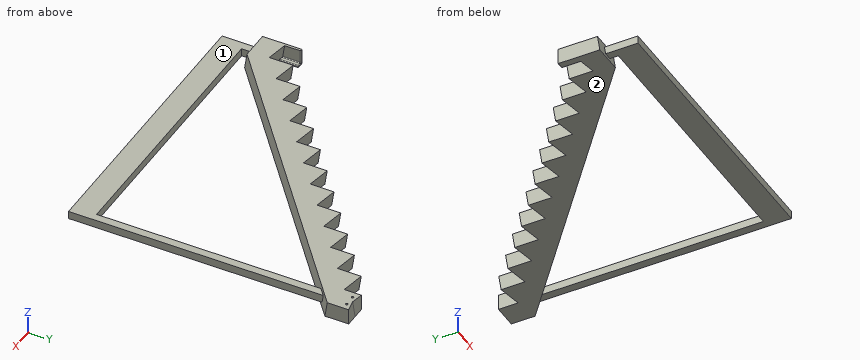
```python
from build123d import *

# Parameters (mm, degrees)
BOSS_EXTRUDE3_DEPTH      = 20
BOSS_EXTRUDE3_DEPTH_BACK = 13
FILLET2_R                = 1
BOSS_EXTRUDE4_DEPTH      = 20
BOSS_EXTRUDE4_DEPTH_BACK = 40
SKETCH10_W               = 10
SKETCH10_H               = 10
BOSS_EXTRUDE5_DEPTH      = 300
BOSS_EXTRUDE5_DEPTH_BACK = 40
SKETCH12_W               = 10
SKETCH12_H               = 10
SKETCH13_W               = 360
SKETCH13_H               = 30
BOSS_EXTRUDE6_DEPTH      = 10
SKETCH14_R               = 1.5
CUT_EXTRUDE1_DEPTH       = 10


with BuildPart() as part:
    # Sketch1 → Loft1 section 0
    with BuildSketch(Plane.XY):
        with BuildLine():
            Line((0, 0), (-30, 5.289809421))
            Line((-30, 5.289809421), (-30, -24.710190579))
            Line((-30, -24.710190579), (-60, -19.420381157))
            Line((-60, -19.420381157), (-60, -49.420381157))
            Line((-60, -49.420381157), (-90, -44.130571736))
            Line((-90, -44.130571736), (-90, -74.130571736))
            Line((-90, -74.130571736), (-120, -68.840762315))
            Line((-120, -68.840762315), (-120, -98.840762315))
            Line((-120, -98.840762315), (-150, -93.550952894))
            Line((-150, -93.550952894), (-150, -123.550952894))
            Line((-150, -123.550952894), (-180, -118.261143472))
            Line((-180, -118.261143472), (-180, -148.261143472))
            Line((-180, -148.261143472), (-210, -142.971334051))
            Line((-210, -142.971334051), (-210, -172.971334051))
            Line((-210, -172.971334051), (-240, -167.68152463))
            Line((-240, -167.68152463), (-240, -197.68152463))
            Line((-240, -197.68152463), (-270, -192.391715209))
            Line((-270, -192.391715209), (-270, -222.391715209))
            Line((-270, -222.391715209), (-300, -217.101905787))
            Line((-300, -217.101905787), (-300, -247.101905787))
            Line((-300, -247.101905787), (-330, -241.812096366))
            Line((-330, -241.812096366), (-330, -271.812096366))
            Line((-330, -271.812096366), (-360, -266.522286945))
            Line((-360, -266.522286945), (-360, -296.522286945))
            Line((-360, -296.522286945), (-390, -291.232477524))
            Line((-390, -291.232477524), (-390, -321.232477524))
            Line((-390, -321.232477524), (-353.577779899, -321.232477524))
            Line((-353.577779899, -321.232477524), (0, -30))
            Line((0, -30), (0, 0))
        make_face()
    # Sketch2 → Loft1 section 1
    with BuildSketch(Plane.XY.offset(-20)):
        with BuildLine():
            Line((-353.577779899, -324.232477524), (-390, -324.232477524))
            Line((-390, -324.232477524), (-390, -294.232477524))
            Line((-390, -294.232477524), (-360, -299.522286945))
            Line((-360, -299.522286945), (-360, -269.522286945))
            Line((-360, -269.522286945), (-330, -274.812096366))
            Line((-330, -274.812096366), (-330, -244.812096366))
            Line((-330, -244.812096366), (-300, -250.101905787))
            Line((-300, -250.101905787), (-300, -220.101905787))
            Line((-300, -220.101905787), (-270, -225.391715209))
            Line((-270, -225.391715209), (-270, -195.391715209))
            Line((-270, -195.391715209), (-240, -200.68152463))
            Line((-240, -200.68152463), (-240, -170.68152463))
            Line((-240, -170.68152463), (-210, -175.971334051))
            Line((-210, -175.971334051), (-210, -145.971334051))
            Line((-210, -145.971334051), (-180, -151.261143472))
            Line((-180, -151.261143472), (-180, -121.261143472))
            Line((-180, -121.261143472), (-150, -126.550952894))
            Line((-150, -126.550952894), (-150, -96.550952894))
            Line((-150, -96.550952894), (-120, -101.840762315))
            Line((-120, -101.840762315), (-120, -71.840762315))
            Line((-120, -71.840762315), (-90, -77.130571736))
            Line((-90, -77.130571736), (-90, -47.130571736))
            Line((-90, -47.130571736), (-60, -52.420381157))
            Line((-60, -52.420381157), (-60, -22.420381157))
            Line((-60, -22.420381157), (-30, -27.710190579))
            Line((-30, -27.710190579), (-30, 2.289809421))
            Line((-30, 2.289809421), (0, -3))
            Line((0, -3), (0, -33))
            Line((0, -33), (-353.577779899, -324.232477524))
        make_face()
    loft()

    # Sketch8 → Cut-Loft1 section 0
    with BuildSketch(Plane(origin=(0, 0, -20), x_dir=(-1, 0, 0), z_dir=(0, 0, -1))):
        with BuildLine():
            Line((0, -3), (30, -3))
            Line((30, -3), (30, 5.289809421))
            Line((30, 5.289809421), (0, 5.289809421))
            Line((0, 5.289809421), (0, -3))
        make_face()
    # Sketch7 → Cut-Loft1 section 1
    with BuildSketch(Plane.XY):
        with BuildLine():
            Line((0, 5.289809421), (-30, 5.289809421))
            Line((-30, 5.289809421), (-30, -3))
            Line((-30, -3), (-15, -6))
            Line((-15, -6), (0, -3))
            Line((0, -3), (0, 5.289809421))
        make_face()
    loft(mode=Mode.SUBTRACT)

    # Sketch9 → Boss-Extrude3 (add, two sides: drawn at the far end of the back side and taken through both)
    with BuildSketch(Plane(origin=(0, -291.232477524, 0), x_dir=(1, 0, 0), z_dir=(0, 1, 0)).offset(-BOSS_EXTRUDE3_DEPTH_BACK)):
        Polygon((-390, 0), (-390, 20), (-381, 20), (-381, 17), (-387, 17), (-387, 0), align=None)
    extrude(amount=BOSS_EXTRUDE3_DEPTH + BOSS_EXTRUDE3_DEPTH_BACK)

    # Fillet2
    fillet2_edges = [part.edges().sort_by_distance(p)[0] for p in [
        (-387, -271.232477524, -8.5),
        (-385.5, -271.232477524, -20),
        (-384, -271.232477524, -17),
        (-381, -283.525948937, -20),
        (-381, -283.300948937, -17),
        (-387, -282.771967995, -17),
    ]]
    fillet(fillet2_edges, radius=FILLET2_R)

    # Sketch12 → Boss-Extrude5 (add, two sides: drawn at the far end of the back side and taken through both)
    with BuildSketch(Plane(origin=(0, -324.232477524, 0), x_dir=(1, 0, 0), z_dir=(0, 1, 0)).offset(-BOSS_EXTRUDE5_DEPTH_BACK)):
        with Locations((-20, 10)):
            Rectangle(SKETCH12_W, SKETCH12_H)
    extrude(amount=BOSS_EXTRUDE5_DEPTH + BOSS_EXTRUDE5_DEPTH_BACK)



with BuildPart() as body_2:
    # Sketch10 → Boss-Extrude4 (new, two sides: drawn at the far end of the back side and taken through both)
    with BuildSketch(Plane(origin=(0, -324.232477524, 0), x_dir=(1, 0, 0), z_dir=(0, 1, 0)).offset(-BOSS_EXTRUDE4_DEPTH_BACK)):
        with Locations((-370, 10)):
            Rectangle(SKETCH10_W, SKETCH10_H)
    extrude(amount=BOSS_EXTRUDE4_DEPTH + BOSS_EXTRUDE4_DEPTH_BACK)


with BuildPart() as part_1:
    add(part.part)

    add(body_2.part)  # Boss-Extrude6 merges body 2
    # Sketch13 → Boss-Extrude6 (add)
    with BuildSketch(Plane(origin=(0, 0, -15), x_dir=(-1, 0, 0), z_dir=(0, 0, -1))):
        with Locations((195, -349.232477524)):
            Rectangle(SKETCH13_W, SKETCH13_H)
    extrude(amount=-BOSS_EXTRUDE6_DEPTH)

    # Sketch14 → Cut-Extrude1 (cut)
    with BuildSketch(Plane.XY):
        with Locations((-22, -9.855095289)):
            Circle(SKETCH14_R)
        with Locations((-8, -9.855095289)):
            Circle(SKETCH14_R)
    extrude(amount=-CUT_EXTRUDE1_DEPTH, mode=Mode.SUBTRACT)


solid = part_1.part
```
Geometry: final body of the model. Coordinates: model frame, mm. Face numbers are marked on the shaded views. A direction names the side the tool comes from. Coordinates: 2 decimals unless noted, no trailing zeros. Write item = value, one per line.
(1) Pin query (flat end, axial travel): pin 1 Ø1.5 at (x, y) = (-21.5, -9.5) entering from +Z; pin 2 Ø5 at (y, z) = (-326, -11) entering from +X; pin 3 Ø0.8 at (y, z) = (-281.5, -18.5) entering from +X. Return the tip coordinate at first contact, or that it passes through.
Solved:
pin_1 = -10
pin_2 = -15
pin_3 = -301.48
(2) Line query: line 1 (X direction, y = -204.5, z = -10.75); line 2 (Y direction, x = -134, z = -11.25); line 3 (Y direction, x = -139, z = -12.25). Output: solid intervals per line, ascending.
Solved:
line_1 = -270 to -209.9, -25 to -15
line_2 = -364.23 to -334.23, -142.06 to -98.06
line_3 = -364.23 to -334.23, -146.33 to -97.33
(3) Access query for the marked faces 1 and 2. Directions: +Z, -Z, +X, -X, +Y, -Y. A direction counts if a zero-diameter tool reaches every point of the face in a straight line with its end or side. Return the directions, or none.
Solved:
face_1 = +Z, +X, -Y
face_2 = -Z, +X, -X, +Y, -Y
